Source: CAD feature listing. Evaluate the final solid. Frame: model axes, mm. A direction names the side the tool comes from. Give positions to 0.01 mm unless a question says otherwise; leave off trailing zeros. Loops run counter-clockwise (first coordinate to the right, second up) from the corner with the lowest first, then second, coordinate; pieces in that order, holes last. Notation, with made-up numbers: M 80.5,5.5 L 119.5,5.5 A17 ccw 119.5,19.5 Z; hole C -2,-5 d4. An arc over 180 degrees is marked long. Answer in a Markdown table with one row per item.
```python
from build123d import *

# Parameters (mm, degrees)
SKETCH1_R           = 50
SKETCH1_R_2         = 3.55
BOSS_EXTRUDE1_DEPTH = 5
SKETCH1_3_R         = 3.55
SKETCH1_3_R_2       = 1.55
BOSS_EXTRUDE2_DEPTH = 2
SKETCH2_R           = 5.5
CUT_EXTRUDE1_DEPTH  = 2.5
CUT_EXTRUDE2_DEPTH  = 10


with BuildPart() as part:
    # Sketch1 → Boss-Extrude1 (new body)
    with BuildSketch(Plane(origin=(0, 0, 0), x_dir=(1, 0, 0), z_dir=(0, 1, 0))):
        with Locations(Location((0, 0, 0), (0, 0, 270))):
            Circle(SKETCH1_R)
        with Locations(Location((25.355339059, -25.355339059, 0), (0, 0, 270))):
            Circle(SKETCH1_R_2, mode=Mode.SUBTRACT)
        with Locations(Location((25.355339059, 25.355339059, 0), (0, 0, 270))):
            Circle(SKETCH1_R_2, mode=Mode.SUBTRACT)
        with Locations(Location((-25.355339059, 25.355339059, 0), (0, 0, 270))):
            Circle(SKETCH1_R_2, mode=Mode.SUBTRACT)
        with Locations(Location((-25.355339059, -25.355339059, 0), (0, 0, 270))):
            Circle(SKETCH1_R_2, mode=Mode.SUBTRACT)
    extrude(amount=BOSS_EXTRUDE1_DEPTH)

    # Sketch1_3 → Boss-Extrude2 (add)
    # profile 1 of 4: a face of its own
    with BuildSketch(Plane(origin=(0, 0, 0), x_dir=(1, 0, 0), z_dir=(0, 1, 0))):
        with Locations(Location((25.355339059, -25.355339059, 0), (0, 0, 270))):
            Circle(SKETCH1_3_R)
        with Locations(Location((25.355339059, -25.355339059, 0), (0, 0, 270))):
            Circle(SKETCH1_3_R_2, mode=Mode.SUBTRACT)
    # profile 2 of 4: a face of its own
    with BuildSketch(Plane(origin=(0, 0, 0), x_dir=(1, 0, 0), z_dir=(0, 1, 0))):
        with Locations(Location((25.355339059, 25.355339059, 0), (0, 0, 270))):
            Circle(SKETCH1_3_R)
        with Locations(Location((25.355339059, 25.355339059, 0), (0, 0, 270))):
            Circle(SKETCH1_3_R_2, mode=Mode.SUBTRACT)
    # profile 3 of 4: a face of its own
    with BuildSketch(Plane(origin=(0, 0, 0), x_dir=(1, 0, 0), z_dir=(0, 1, 0))):
        with Locations(Location((-25.355339059, 25.355339059, 0), (0, 0, 270))):
            Circle(SKETCH1_3_R)
        with Locations(Location((-25.355339059, 25.355339059, 0), (0, 0, 270))):
            Circle(SKETCH1_3_R_2, mode=Mode.SUBTRACT)
    # profile 4 of 4: a face of its own
    with BuildSketch(Plane(origin=(0, 0, 0), x_dir=(1, 0, 0), z_dir=(0, 1, 0))):
        with Locations(Location((-25.355339059, -25.355339059, 0), (0, 0, 270))):
            Circle(SKETCH1_3_R)
        with Locations(Location((-25.355339059, -25.355339059, 0), (0, 0, 270))):
            Circle(SKETCH1_3_R_2, mode=Mode.SUBTRACT)
    extrude(amount=BOSS_EXTRUDE2_DEPTH)

    # Sketch2 → Cut-Extrude1 (cut)
    with BuildSketch(Plane.XZ):
        with Locations(Location((0, 35.355339059, 0), (0, 0, 270))):
            Circle(SKETCH2_R)
    extrude(amount=-CUT_EXTRUDE1_DEPTH, mode=Mode.SUBTRACT)

    # Sketch3 → Cut-Extrude2 (cut)
    with BuildSketch(Plane(origin=(0, 5, 0), x_dir=(1, 0, 0), z_dir=(0, 1, 0))):
        Polygon((0, 28.867513459), (-25, 14.43375673), (-25, -14.43375673), (0, -28.867513459), (25, -14.43375673), (25, 14.43375673), align=None)
    extrude(amount=-CUT_EXTRUDE2_DEPTH, mode=Mode.SUBTRACT)


solid = part.part
```
1) Section C-C, the plane y = 1.05. Return loops of the section in (x, z), then the cut area to 3 significant figures.
Reply:
| item | result |
|---|---|
| outline | C 0,0 d100; hole C -25.36,-25.36 d3.1; hole C -25.36,25.36 d3.1; hole M -25,-14.43 L 0,-28.87 L 25,-14.43 L 25,14.43 L 0,28.87 L -25,14.43 Z; hole C 0,35.36 d11; hole C 25.36,-25.36 d3.1; hole C 25.36,25.36 d3.1 |
| area | 5,560 mm² |
2) Section A-A, the plane z = 0. Return loops of the section in (x, y), then the cut area to 3 significant figures.
Reply:
| item | result |
|---|---|
| outline | M -50,0 L -25,0 L -25,5 L -50,5 Z; M 25,0 L 50,0 L 50,5 L 25,5 Z |
| area | 250 mm² |
3) Section B-B, the plane x = 20. Return loops of the section in (y, z).
Reply:
| item | result |
|---|---|
| outline | M 0,-45.83 L 5,-45.83 L 5,-17.32 L 0,-17.32 Z; M 0,17.32 L 5,17.32 L 5,45.83 L 0,45.83 Z |
4) Pin query (flat end, axial travel): pin 1 Ø6.5 at (x, z) = (25.36, -25.36) entering from +Y; pin 2 Ø1 at (y, z) = (3.5, -9.5) entering from -X; pin 3 Ø3.5 at (x, z) = (-2, 34) entering from -Y. Return the tip coordinate at first contact, or that it passes through.
Reply:
| item | result |
|---|---|
| pin 1 | stops at y = 2 |
| pin 2 | stops at x = -49.18 |
| pin 3 | stops at y = 2.5 |
5) Section D-D, the plane z = 44.5. Return loops of the section in (x, y).
Reply:
| item | result |
|---|---|
| outline | M -22.8,0 L 22.8,0 L 22.8,5 L -22.8,5 Z |
6) Pull-direction query (Z, two-part tool) for faces 1 (the cylindrical face through (15.02, 2.46, 47.69)), 2 (the flat face through (12, 0, -23)), 3 (the cylindrical face through (24.412, 0.986, 24.125)), 4 (the flat face through (-25, 3, 0)); classes: released by +Z, released by -Z, zero draft, split by the parting line, or undercut.
Reply:
| item | result |
|---|---|
| face 1 | split by the parting line |
| face 2 | zero draft |
| face 3 | undercut |
| face 4 | undercut |
7) Set-up query: faces 5 (the flat face through (12, 5, -23)), 6 (the flat face through (0, 2.5, 35)), 7 (the flat face through (-12.675, 2.535, 21.55)), 8 (the cylindrical face through (-23, 3.5, 22.7)). Return all of +Z, -Z, +X, -X, +Y, -Y with unobstructed straight access to the full face (end or side cutting, diameter ignored); none if empty.
Reply:
| item | result |
|---|---|
| face 5 | +Z, -Z, +X, -X, +Y |
| face 6 | -Y |
| face 7 | +Y, -Y |
| face 8 | +Y |
8) Material intervals for L1, parallel to Z at x = 24.5, y = 1.1; L2, parallel to Z at x = 5, y = 1.2; L3, parallel to Z at x = 27.5, y = 3.2, sorted ascending.
Reply:
| item | result |
|---|---|
| L1 | z = -43.59 to -26.65, -24.06 to -14.72, 14.72 to 24.06, 26.65 to 43.59 |
| L2 | z = -49.75 to -25.98, 25.98 to 33.06, 37.65 to 49.75 |
| L3 | z = -41.76 to -28.18, -22.53 to 22.53, 28.18 to 41.76 |
